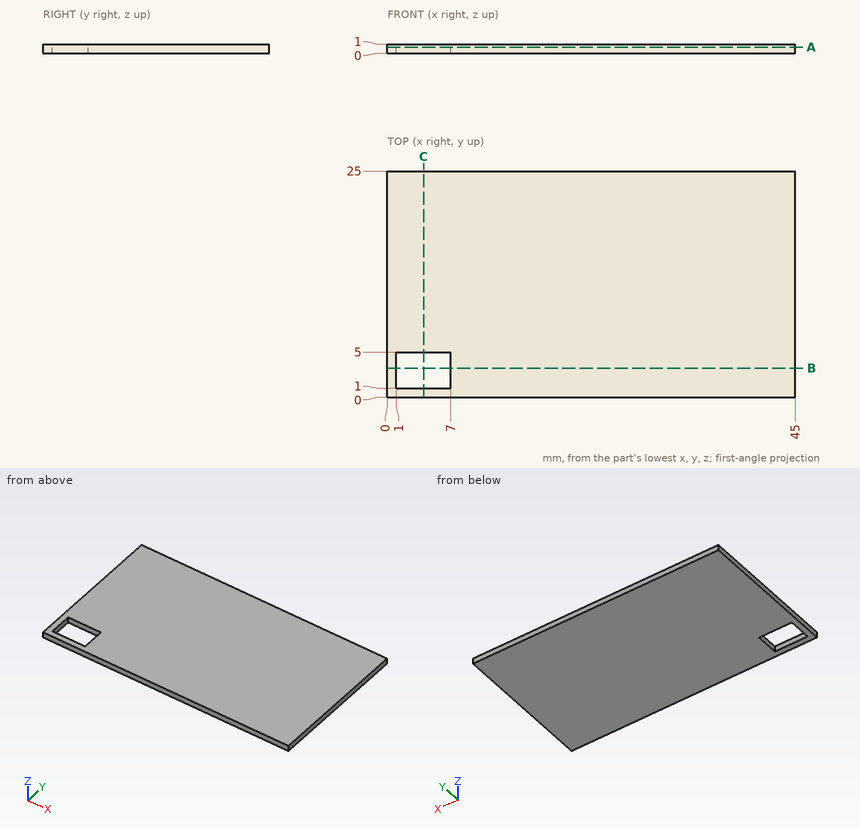
Study the drawing (mm; zero at the part's minimum x, y, z) and answer. Give positions to 0.01 mm unless a question says otherwise; leave off trailing zeros. Order: outer loops, then holes, each group sorted by start corner. A loop starts at its lowest first (then second) coordinate and runs counter-clockwise, first axis right, second up.
1) Find section C-C on x = 4. Write down the section's boundary in (y, z).
Reported:
outline: (0, 0) - (1, 0) - (1, 1) - (0, 1) - close; (5, 0) - (25, 0) - (25, 1) - (5, 1) - close
2) Find section B-B on y = 3.25. Write down the section's boundary in (x, z), then the cut area to 3 significant figures.
Reported:
outline: (0, 0) - (1, 0) - (1, 1) - (0, 1) - close; (7, 0) - (45, 0) - (45, 1) - (7, 1) - close
area: 39.0 mm2
3) Consider line 1 along X through (y, z) = (1.5, 0.5). Determine where the line is inside the solid, lowest interval first.
Reported:
line 1: x = 0 to 1, 7 to 45
4) Find section A-A on z = 0.65. Write down the section's boundary in (x, y), then the cut area to 3 significant figures.
Reported:
outline: (0, 0) - (45, 0) - (45, 25) - (0, 25) - close; hole (1, 1) - (7, 1) - (7, 5) - (1, 5) - close
area: 1,100 mm2
5) Given P1, Ø0.5, axis at y = 2.5, z = 0.5, coming from the -X side, flat-ended and moving along its own axis, determine where the tip first touches the part or whether it passes through.
Reported:
P1: stops at x = 0
